Verification items for the finished model (mm, model axes). Face numbers are marked on the shaded views. Round coordinates to 2 decimals unless told otherwise and drop trailing zeros. Order: outer loops, then holes, each group sorted by start corner. A loop starts at its lowest first (then second) coordinate and runs counter-clockwise, first axis right, second up. Notation, with made-up numbers: M -2,9.5 L 47,9.5 A29 ccw 47,39.5 Z; hole C 57,18.25 d4. An arc over 180 degrees is marked long. Return JSON: item names as keys, results as strings. Group by question number.
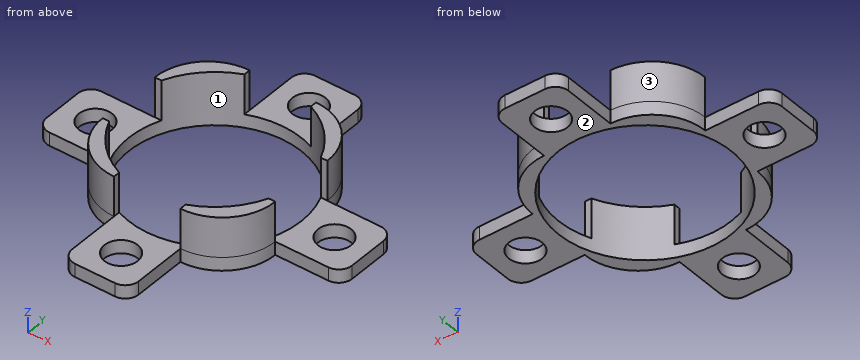
Autodesk Inventor part; units mm, degrees
ref_plane "Work Plane1" through (82.85, -94.2541, 8) normal (0, 0, 1) x (1, 0, 0)
ref_plane "Work Plane2" through (82.85, -94.2541, 8) normal (0, 0, 1) x (1, 0, 0)
ref_plane "YZ Plane" through (0, 0, 0) normal (1, 0, 0) x (0, 1, 0)
sketch "Sketch1" plane through (0, 0, 0) normal (0, 0, 1) x (1, 0, 0)
  circle A0 centre (95.85, -81.2541) radius 13
  line L0 (108.85, -68.2541) -> (108.85, -94.2541)
  line L1 (82.85, -94.2541) -> (82.85, -68.2541)
  line L2 (82.85, -68.2541) -> (108.85, -68.2541)
  line L3 (82.85, -81.2541) -> (77.85, -81.2541) construction
  line L4 (95.85, -68.2541) -> (95.85, -63.2541) construction
  line L5 (108.85, -81.2541) -> (113.85, -81.2541) construction
  line L6 (108.85, -81.2541) -> (113.85, -81.2541) construction
  line L7 (95.85, -94.2541) -> (95.85, -99.2541) construction
  line L8 (92.85, -58.2541) -> (98.85, -58.2541)
  line L9 (100.85, -60.2541) -> (100.85, -68.2541)
  line L10 (100.85, -68.2541) -> (90.85, -68.2541)
  line L11 (90.85, -68.2541) -> (90.85, -60.2541)
  line L12 (90.85, -58.2541) -> (100.85, -68.2541) construction
  line L13 (100.85, -58.2541) -> (90.85, -68.2541) construction
  line L14 (116.85, -76.2541) -> (108.85, -76.2541)
  line L15 (108.85, -76.2541) -> (108.85, -86.2541)
  line L16 (108.85, -86.2541) -> (116.85, -86.2541)
  line L17 (118.85, -84.2541) -> (118.85, -78.2541)
  line L18 (118.85, -76.2541) -> (108.85, -86.2541) construction
  line L19 (108.85, -76.2541) -> (118.85, -86.2541) construction
  line L20 (92.85, -104.2541) -> (98.85, -104.2541)
  line L21 (100.85, -102.2541) -> (100.85, -94.2541)
  line L22 (95.85, -94.2541) -> (90.85, -94.2541)
  line L23 (90.85, -94.2541) -> (90.85, -102.2541)
  line L24 (90.85, -104.2541) -> (100.85, -94.2541) construction
  line L25 (100.85, -104.2541) -> (90.85, -94.2541) construction
  line L26 (74.85, -86.2541) -> (82.85, -86.2541)
  line L27 (82.85, -86.2541) -> (82.85, -76.2541)
  line L28 (82.85, -76.2541) -> (74.85, -76.2541)
  line L29 (72.85, -78.2541) -> (72.85, -84.2541)
  line L30 (72.85, -86.2541) -> (82.85, -76.2541) construction
  line L31 (82.85, -86.2541) -> (72.85, -76.2541) construction
  circle A1 centre (77.85, -81.2541) radius 2.5
  circle A2 centre (95.85, -63.2541) radius 2.5
  circle A3 centre (113.85, -81.2541) radius 2.5
  circle A4 centre (95.85, -99.2541) radius 2.5
  line L32 (108.85, -94.2541) -> (95.85, -94.2541)
  line L33 (90.85, -94.2541) -> (82.85, -94.2541)
  arc A5 (92.85, -58.2541) -> (90.85, -60.2541) centre (92.85, -60.2541) ccw
  arc A6 (100.85, -60.2541) -> (98.85, -58.2541) centre (98.85, -60.2541) ccw
  arc A7 (118.85, -78.2541) -> (116.85, -76.2541) centre (116.85, -78.2541) ccw
  arc A8 (116.85, -86.2541) -> (118.85, -84.2541) centre (116.85, -84.2541) ccw
  arc A9 (98.85, -104.2541) -> (100.85, -102.2541) centre (98.85, -102.2541) ccw
  arc A10 (90.85, -102.2541) -> (92.85, -104.2541) centre (92.85, -102.2541) ccw
  arc A11 (72.85, -84.2541) -> (74.85, -86.2541) centre (74.85, -84.2541) ccw
  arc A12 (74.85, -76.2541) -> (72.85, -78.2541) centre (74.85, -78.2541) ccw
  point P0 (0, 0)
  dimension "d0" = 5
  dimension "d1" = 5
  dimension "d2" = 5
  dimension "d3" = 0
  dimension "d4" = 5
  dimension "d5" = 10
  dimension "d6" = 5
  dimension "d7" = 5
  dimension "d8" = 5
  dimension "d9" = 5
  dimension "d10" = 2
ref_plane "Work Plane1" through (82.85, -94.2541, 8) normal (0, 0, 1) x (1, 0, 0)
extrude "Extrusion1" add sketch "Sketch1" along normal blind 2 contours L22 L33 L1 A0 | L32 L21 A9 L20 A10 L23 L22 | A0 L0 L32 | A0 L2 L0 | L0 L14 A7 L17 A8 L16 | L1 L2 A0 | L1 L26 A11 L29 A12 L28 | L2 L11 A5 L8 A6 L9
fillet "Fillet1" radius 8 4 edges at (108.85, -68.2541, 1) (82.85, -68.2541, 1) (82.85, -94.2541, 1) (108.85, -94.2541, 1)
sketch "Sketch2" plane through (0, 0, 2) normal (0, 0, 1) x (1, 0, 0)
  arc A0 (100.85, -94.2541) -> (108.85, -86.2541) centre (100.85, -86.2541) ccw
  line L0 (108.85, -86.2541) -> (116.85, -86.2541)
  arc A1 (116.85, -86.2541) -> (118.85, -84.2541) centre (116.85, -84.2541) ccw
  line L1 (118.85, -84.2541) -> (118.85, -78.2541)
  arc A2 (118.85, -78.2541) -> (116.85, -76.2541) centre (116.85, -78.2541) ccw
  line L2 (116.85, -76.2541) -> (108.85, -76.2541)
  arc A3 (108.85, -76.2541) -> (100.85, -68.2541) centre (100.85, -76.2541) ccw
  line L3 (100.85, -68.2541) -> (100.85, -60.2541)
  arc A4 (100.85, -60.2541) -> (98.85, -58.2541) centre (98.85, -60.2541) ccw
  line L4 (98.85, -58.2541) -> (92.85, -58.2541)
  arc A5 (92.85, -58.2541) -> (90.85, -60.2541) centre (92.85, -60.2541) ccw
  line L5 (90.85, -60.2541) -> (90.85, -68.2541)
  arc A6 (90.85, -68.2541) -> (82.85, -76.2541) centre (90.85, -76.2541) ccw
  line L6 (82.85, -76.2541) -> (74.85, -76.2541)
  arc A7 (74.85, -76.2541) -> (72.85, -78.2541) centre (74.85, -78.2541) ccw
  line L7 (72.85, -78.2541) -> (72.85, -84.2541)
  arc A8 (72.85, -84.2541) -> (74.85, -86.2541) centre (74.85, -84.2541) ccw
  line L8 (74.85, -86.2541) -> (82.85, -86.2541)
  arc A9 (82.85, -86.2541) -> (90.85, -94.2541) centre (90.85, -86.2541) ccw
  line L9 (90.85, -94.2541) -> (90.85, -102.2541)
  arc A10 (90.85, -102.2541) -> (92.85, -104.2541) centre (92.85, -102.2541) ccw
  line L10 (92.85, -104.2541) -> (98.85, -104.2541)
  arc A11 (98.85, -104.2541) -> (100.85, -102.2541) centre (98.85, -102.2541) ccw
  line L11 (100.85, -102.2541) -> (100.85, -94.2541)
  circle A12 centre (95.85, -99.2541) radius 2.5
  circle A13 centre (113.85, -81.2541) radius 2.5
  circle A14 centre (95.85, -63.2541) radius 2.5
  circle A15 centre (77.85, -81.2541) radius 2.5
  circle A16 centre (95.85, -81.2541) radius 13
  line L12 (90.85, -68.2541) -> (90.85, -69.2541)
  line L13 (100.85, -68.2541) -> (100.85, -69.2541)
  line L14 (108.85, -76.2541) -> (107.85, -76.2541)
  line L15 (108.85, -86.2541) -> (107.85, -86.2541)
  line L16 (100.85, -94.2541) -> (100.85, -93.2541)
  line L17 (90.85, -94.2541) -> (90.85, -93.2541)
  line L18 (82.85, -86.2541) -> (83.85, -86.2541)
  line L19 (82.85, -76.2541) -> (83.85, -76.2541)
  circle A17 centre (95.85, -81.2541) radius 13
  point P0 (0, 0)
ref_plane "Work Plane2" through (82.85, -94.2541, 8) normal (0, 0, 1) x (1, 0, 0)
extrude "Extrusion2" add sketch "Sketch2" along normal up to surface (6 mm away) contours L16 A16 L15 A0 | L17 A9 L18 A16 | A16 L13 A3 L14 | L19 A6 L12 A16
properties part number "BearingMountMK2"
1. Cross-section at C-C (x = 95.85). Enter the section's corners in (y, z), plus the area to 3 significant figures.
2. Draft check along Y on the marked faces 1, 2 and 3. Enter one of: +Y half, -Y half, draft (parallel to the pull), parting line (faces both ways), or undercut.
3. Cross-section at B-B (z = 3). Enter the section's corners in (x, y), plus the area to 3 significant figures.
4. Cross-section at A-A (x = 113.85). Enter the section's corners in (y, z), plus the area to 3 significant figures.
5. Go/stop test with flat-tipped pins: pin 1 (1.5 mm diameter, centred on y = -70.5, z = 3, fed in from +X); pin 2 (1.1 mm diameter, centred on x = 83.5, z = 5.5, fed in from -Y); pin 3 (0.6 mm diameter, centred on x = 114.5, z = 1, fed in from +Y); pin 4 (3 mm diameter, centred on y = -96.5, z = 4.5, fed in from +X). Record where each tip stops, or that it passes through.
6. Cross-section at D-D (y = -100). Enter the section's corners in (x, z), plus the area to 3 significant figures.
7. Thickness scan on line 1 along Y through (x, z) = (95.85, 1.15); line 2 along Y through (x, z) = (87, 7.75); line 3 along X through (y, z) = (-71, 4). Record the ranges inside material, lowest first. Write a range as from..to.
Computed:
{
 "1": {"outline": "M -104.25,0 L -101.75,0 L -101.75,2 L -104.25,2 Z; M -96.75,0 L -94.25,0 L -94.25,2 L -96.75,2 Z; M -68.25,0 L -65.75,0 L -65.75,2 L -68.25,2 Z; M -60.75,0 L -58.25,0 L -58.25,2 L -60.75,2 Z", "area": "20.0 mm²"},
 "2": {"face 1": "undercut", "face 2": "draft", "face 3": "+Y half"},
 "3": {"outline": "M 82.85,-86.25 A8 ccw 90.85,-94.25 L 90.85,-93.25 A13 cw 83.85,-86.25 Z; M 82.85,-76.25 L 83.85,-76.25 A13 cw 90.85,-69.25 L 90.85,-68.25 A8 ccw Z; M 100.85,-94.25 A8 ccw 108.85,-86.25 L 107.85,-86.25 A13 cw 100.85,-93.25 Z; M 100.85,-69.25 A13 cw 107.85,-76.25 L 108.85,-76.25 A8 ccw 100.85,-68.25 Z", "area": "77.0 mm²"},
 "4": {"outline": "M -86.25,0 L -83.75,0 L -83.75,2 L -86.25,2 Z; M -78.75,0 L -76.25,0 L -76.25,2 L -78.75,2 Z", "area": "10.0 mm²"},
 "5": {"pin 1": "stops at x = 107.09", "pin 2": "stops at y = -90.47", "pin 3": "stops at y = -76.25", "pin 4": "passes through"},
 "6": {"outline": "M 90.85,0 L 93.46,0 L 93.46,2 L 90.85,2 Z; M 98.24,0 L 100.85,0 L 100.85,2 L 98.24,2 Z", "area": "10.5 mm²"},
 "7": {"line 1": "y = -104.25..-101.75, -96.75..-94.25, -68.25..-65.75, -60.75..-58.25", "line 2": "y = -93.27..-90.78, -71.73..-69.24", "line 3": "x = 84.82..87.86, 103.84..106.88"}
}
